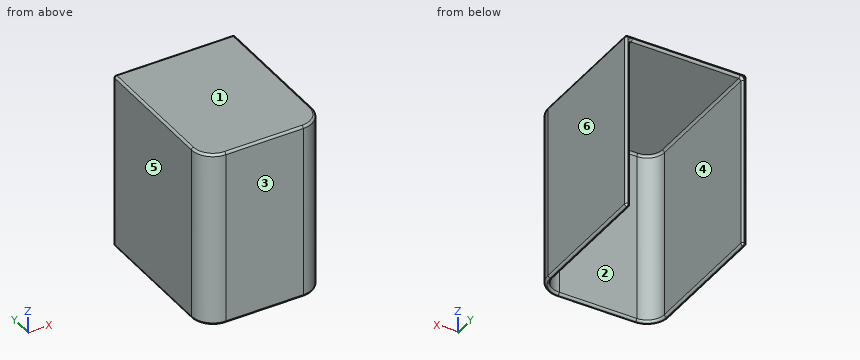
```python
from build123d import *

# Parameters (mm, degrees)
F1_DEPTH = 254
F3_DEPTH = 6.35
F4_F1_R  = 3.175
F4_F2_R  = 3.1749


# Not quite as in the source:
# - a fillet or chamfer is up to 0.001 mm smaller than in the source, because OpenCascade refuses the exact size


with BuildPart() as f1:
    # F0 (on Top) → F1 (new body)
    with BuildSketch(Plane.XY):
        with BuildLine():
            Line((57.15, -215.9), (-57.15, -215.9))
            ThreePointArc((-57.15, -215.9), (-75.1105122421, -208.4605122421), (-82.55, -190.5))
            Line((-82.55, -190.5), (-82.55, 0))
            Line((-82.55, 0), (-88.9, 0))
            Line((-88.9, 0), (-88.9, -190.5))
            ThreePointArc((-88.9, -190.5), (-79.6006403027, -212.9506403027), (-57.15, -222.25))
            Line((-57.15, -222.25), (57.15, -222.25))
            ThreePointArc((57.15, -222.25), (79.6006403027, -212.9506403027), (88.9, -190.5))
            Line((88.9, -190.5), (88.9, 0))
            Line((88.9, 0), (82.55, 0))
            Line((82.55, 0), (82.55, -190.5))
            ThreePointArc((82.55, -190.5), (75.1105122421, -208.4605122421), (57.15, -215.9))
        make_face()
    extrude(amount=F1_DEPTH)

    # F2 (on face) → F3 (join)
    with BuildSketch(Plane.XY.offset(254)):
        with BuildLine():
            Line((82.55, 0), (-82.55, 0))
            Line((-82.55, 0), (-82.55, -190.5))
            ThreePointArc((-82.55, -190.5), (-75.1105122421, -208.4605122421), (-57.15, -215.9))
            Line((-57.15, -215.9), (57.15, -215.9))
            ThreePointArc((57.15, -215.9), (75.1105122421, -208.4605122421), (82.55, -190.5))
            Line((82.55, -190.5), (82.55, 0))
        make_face()
        with BuildLine():
            Line((-82.55, 0), (-88.9, 0))
            Line((-88.9, 0), (-88.9, -190.5))
            ThreePointArc((-88.9, -190.5), (-79.6006403027, -212.9506403027), (-57.15, -222.25))
            Line((-57.15, -222.25), (57.15, -222.25))
            ThreePointArc((57.15, -222.25), (79.6006403027, -212.9506403027), (88.9, -190.5))
            Line((88.9, -190.5), (88.9, 0))
            Line((88.9, 0), (82.55, 0))
            Line((82.55, 0), (82.55, -190.5))
            ThreePointArc((82.55, -190.5), (75.1105122421, -208.4605122421), (57.15, -215.9))
            Line((57.15, -215.9), (-57.15, -215.9))
            ThreePointArc((-57.15, -215.9), (-75.1105122421, -208.4605122421), (-82.55, -190.5))
            Line((-82.55, -190.5), (-82.55, 0))
        make_face()
    extrude(amount=F3_DEPTH)

    # F4: fillet of radius 3.175 on 23 edges, made by hand

    # F4_f1
    f4_f1_edges = [f1.edges().sort_by_distance(p)[0] for p in [
        (75.1105122421, -208.4605122421, 254),
        (82.55, -95.25, 254),
        (0, -215.9, 254),
        (-75.1105122421, -208.4605122421, 254),
        (-82.55, -95.25, 254),
    ]]
    fillet(f4_f1_edges, radius=F4_F1_R)

    # F4_f2 (radius 3.175 in the source; OpenCascade refuses exactly that, so slightly less here)
    f4_f2_edges = [f1.edges().sort_by_distance(p)[0] for p in [
        (-88.9, -95.25, 260.35),
        (-79.6006403027, -212.9506403027, 260.35),
        (0, -222.25, 260.35),
        (79.6006403027, -212.9506403027, 260.35),
        (88.9, -95.25, 260.35),
        (0, 0, 260.35),
        (88.9, 0, 130.175),
        (-88.9, 0, 130.175),
        (82.55, 0, 125.4125),
        (-82.55, 0, 125.4125),
        (75.1105122421, -208.4605122421, 0),
        (0, -215.9, 0),
        (-75.1105122421, -208.4605122421, 0),
        (-82.55, -95.25, 0),
        (-85.725, 0, 0),
        (-88.9, -95.25, 0),
        (-79.6006403027, -212.9506403027, 0),
        (0, -222.25, 0),
        (79.6006403027, -212.9506403027, 0),
        (88.9, -95.25, 0),
        (85.725, 0, 0),
        (82.55, -95.25, 0),
        (-81.6200640303, 0, 253.0700640303),
        (81.6200640303, 0, 253.0700640303),
    ]]
    fillet(f4_f2_edges, radius=F4_F2_R)


solid = f1.part
```
Input: part model. Units: mm. Frame: model coordinates. Face numbers are marked on the shaded views. A direction names the side the tool comes from. Give positions to 0.01 mm unless a question says otherwise; leave off trailing zeros. Answer as CSV lines item,"result". Start each with the question number.
1. Line query: L1, parallel to X at y = -162.5, z = 225.5; L2, parallel to Z at x = 43.5, y = -199; L3, parallel to Y at x = -13, z = 188.5. Output: solid intervals per line, ascending.
2. Reachability of the marked faces 1 and 2 from +Z, -Z, +X, -X, +Y, -Y: full face, straight path, thin tool, end or side. Return the list, or none.
3. Pull-direction query (X, two-part tool) for the marked faces 3, 4, 5 and 6; classes: released by +X, released by -X, zero draft, split by the parting line, or undercut.
4. Pin query (flat end, axial travel): P1, Ø1.5, axis at x = 29.5, y = -160, coming from the -Z side. Return the tip coordinate at first contact, or that it passes through.
Computed values:
1,L1,"x = -88.9 to -82.55, 82.55 to 88.9"
1,L2,"z = 254 to 260.35"
1,L3,"y = -222.25 to -215.9"
2,face 1,"+Z, +X, -X, +Y, -Y"
2,face 2,"-Z, +Y"
3,face 3,"zero draft"
3,face 4,"undercut"
3,face 5,"released by -X"
3,face 6,"released by +X"
4,P1,"stops at z = 254"
